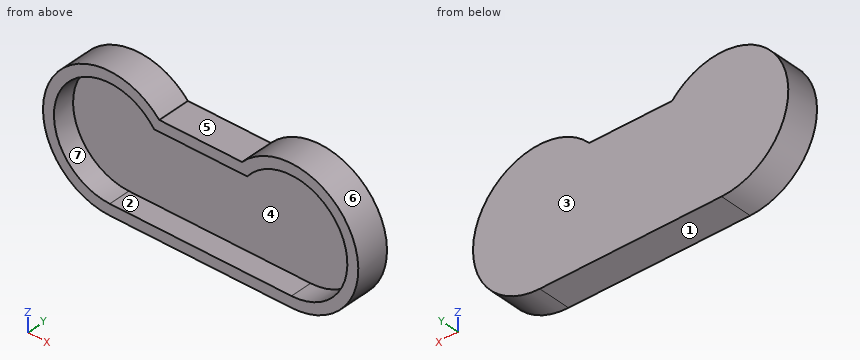
```python
from build123d import *

# Parameters (mm, degrees)
BOSS_EXTRUDE1_DEPTH = 15
CUT_EXTRUDE1_DEPTH  = 10


with BuildPart() as part:
    # Sketch1 → Boss-Extrude1 (new body)
    with BuildSketch(Plane(origin=(0, 0, 0), x_dir=(1, 0, 0), z_dir=(0, 1, 0))):
        with BuildLine():
            Line((41.5, 30.5), (-41.5, 30.5))
            ThreePointArc((-41.5, 30.5), (-69.388169535, -12.349089035), (-18.916820419, -20.5))
            Line((-18.916820419, -20.5), (18.916820419, -20.5))
            ThreePointArc((18.916820419, -20.5), (69.388169535, -12.349089035), (41.5, 30.5))
        make_face()
    extrude(amount=BOSS_EXTRUDE1_DEPTH)

    # Sketch2 → Cut-Extrude1 (cut)
    with BuildSketch(Plane(origin=(0, 0, 0), x_dir=(1, 0, 0), z_dir=(0, 1, 0))):
        with BuildLine():
            Line((41.5, 25.5), (-41.5, 25.5))
            ThreePointArc((-41.5, 25.5), (-64.36372673, -11.291589791), (-21.251543269, -15.5))
            Line((-21.251543269, -15.5), (21.251543269, -15.5))
            ThreePointArc((21.251543269, -15.5), (64.36372673, -11.291589791), (41.5, 25.5))
        make_face()
    extrude(amount=CUT_EXTRUDE1_DEPTH, mode=Mode.SUBTRACT)


solid = part.part
```
Geometry: final body of the model. Coordinates: model frame, mm. Face numbers are marked on the shaded views. A direction names the side the tool comes from. Round coordinates to 2 decimals unless told otherwise and drop trailing zeros. Write each loop counter-clockwise with the first axis right and the second up, starting at its lowest first coordinate (ties: lowest second). Pieces come first, ordered by that corner, then holes.
Item 1: Pin query (flat end, axial travel): P1, Ø8, axis at x = -46.5, y = 7, coming from the -Z side; P2, Ø1, axis at y = 13, z = 1, coming from the -X side; P3, Ø1, axis at x = -40.5, y = 11, coming from the +Z side. Return the tip coordinate at first contact, or that it passes through.
Item 2: Mould query, pull axis Z, two halves, no side actions, for the marked faces 1, 2, 3 and 4. Classes: +Z half, -Z half, draft (parallel to the pull), parting line (faces both ways), or undercut.
Item 3: Material intervals for L1, parallel to X at y = 5.75, z = 0; L2, parallel to Z at x = -41.5, y = 4.25; L3, parallel to Z at x = 2, y = 2.5, sorted ascending.
Item 4: Section query A-A (x = 12.5). Return loops of the section in (y, z), plus the area to 3 significant figures.
Item 5: Section query C-C (y = 11.5). Return loops of the section in (x, z).
Item 6: Section query B-B (z = 4.5). Return loops of the section in (x, y).
Item 7: Section query D-D (z = 24). Return loops of the section in (x, y), plus the area to 3 significant figures.
Item 8: Set-up query: the marked faces 5, 6 and 7. Return all of +Z, -Z, +X, -X, +Y, -Y with unobstructed straight access to the full face (end or side cutting, diameter ignored); none if empty.
Completed:
1. P1: stops at z = -30.48
1. P2: stops at x = -72
1. P3: stops at z = 30.5
2. face 1: -Z half
2. face 2: undercut
2. face 3: draft
2. face 4: undercut
3. L1: x = -72 to -67, 67 to 72
3. L2: z = -30.5 to -25.5, 25.5 to 30.5
3. L3: z = -30.5 to -25.5, 15.5 to 20.5
4. outline: (0, -30.5) - (15, -30.5) - (15, 20.5) - (0, 20.5) - (0, 15.5) - (10, 15.5) - (10, -25.5) - (0, -25.5) - close
4. area: 355 mm2
5. outline: (-41.5, -30.5) - (41.5, -30.5) arc R30.5 ccw (long way) to (18.92, 20.5) - (-18.92, 20.5) arc R30.5 ccw (long way) to start
6. outline: (-71.67, 0) - (-66.6, 0) - (-66.6, 10) - (66.6, 10) - (66.6, 0) - (71.67, 0) - (71.67, 15) - (-71.67, 15) - close
7. outline: (-60.32, 0) - (-50.12, 0) - (-50.12, 10) - (-32.88, 10) - (-32.88, 0) - (-22.68, 0) - (-22.68, 15) - (-60.32, 15) - close; (22.68, 0) - (32.88, 0) - (32.88, 10) - (50.12, 10) - (50.12, 0) - (60.32, 0) - (60.32, 15) - (22.68, 15) - close
7. area: 785 mm2
8. face 5: +Z, +Y, -Y
8. face 6: +Y, -Y
8. face 7: -Y
